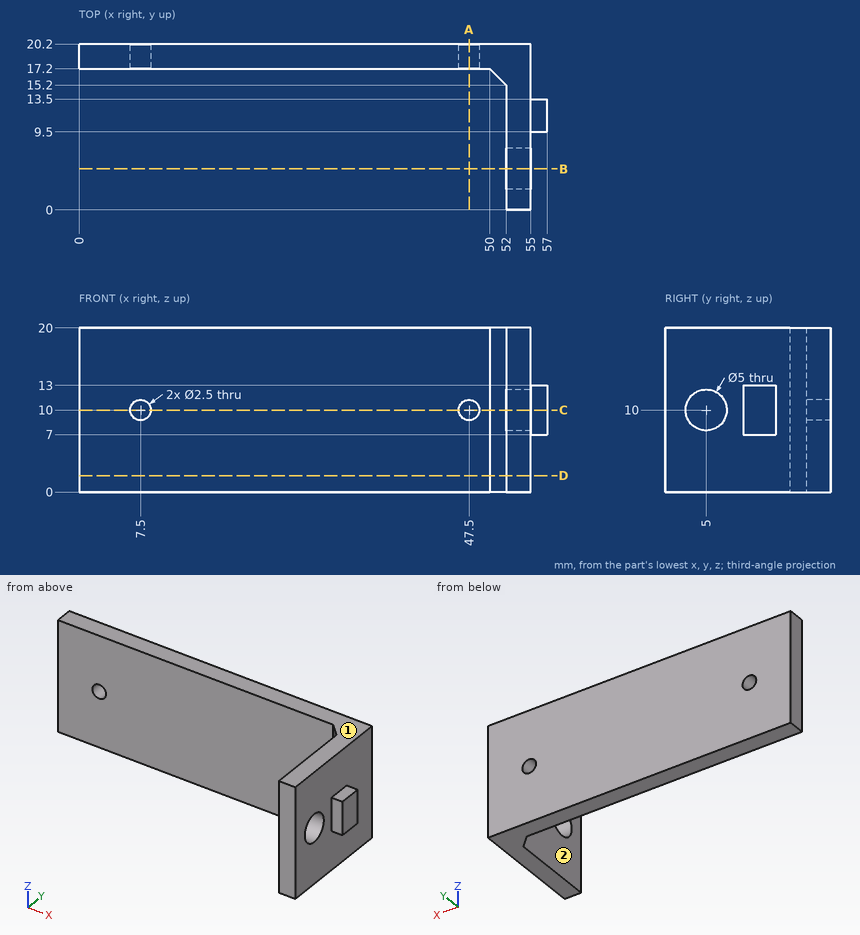
Verification items for this drawing (mm, ordinates from the low corner). A direction names the side the tool comes from. Round coordinates to 2 decimals unless told otherwise and drop trailing zeros. Loops run counter-clockwise (first coordinate to the right, second up) from the corner with the lowest first, then second, coordinate; pieces in that order, holes last. Notation, with made-up numbers: (31.25, 83) -> (78.25, 83) arc R19 cw to (78.25, 111) -> close; hole circle Ø9 at (47, 24.25). An arc over 180 degrees is marked (long way). Answer in a Markdown table with one row per item.
Q1. Go/stop test with flat-tipped pins: P1, Ø3, axis at y = 4.5, z = 5.5, coming from the +X side; P2, Ø0.6, axis at x = 56.5, y = 11.5, coming from the -Z side; P3, Ø0.6, axis at x = 56.5, y = 12.5, coming from the +Z side; P4, Ø1.5, axis at x = 47.5, z = 10, coming from the +Y side. Record where each tip stops, or that it passes through.
Data:
| item | result |
|---|---|
| P1 | stops at x = 55 |
| P2 | stops at z = 7 |
| P3 | stops at z = 13 |
| P4 | passes through |
Q2. Sectioned sample at B-B on y = 5. Enter the section's corners in (x, z), then the cut area to 3 significant figures.
Data:
| item | result |
|---|---|
| outline | (52, 0) -> (55, 0) -> (55, 7.5) -> (52, 7.5) -> close; (52, 12.5) -> (55, 12.5) -> (55, 20) -> (52, 20) -> close |
| area | 45.0 mm^2 |
Q3. Sectioned sample at D-D on z = 2. Enter the section's corners in (x, y), then the cut area to 3 significant figures.
Data:
| item | result |
|---|---|
| outline | (0, 17.2) -> (50, 17.2) -> (52, 15.2) -> (52, 0) -> (55, 0) -> (55, 20.2) -> (0, 20.2) -> close |
| area | 219 mm^2 |
Q4. Set-up check for the marked faces 1 and 2: record each of +Z, -Z, +X, -X, +Y, -Y from which the full face is reachable in a straight line by a thin tool's end or side.
Data:
| item | result |
|---|---|
| face 1 | +Z, +X, -X, +Y, -Y |
| face 2 | +Z, -Z, -X, -Y |
Q5. Sectioned sample at A-A on x = 47.5. Enter the section's corners in (y, z), then the cut area to 3 significant figures.
Data:
| item | result |
|---|---|
| outline | (17.2, 0) -> (20.2, 0) -> (20.2, 8.75) -> (17.2, 8.75) -> close; (17.2, 11.25) -> (20.2, 11.25) -> (20.2, 20) -> (17.2, 20) -> close |
| area | 52.5 mm^2 |
Q6. Thickness scan on L1, parallel to Y at x = 54.05, z = 10; L2, parallel to Z at x = 47.5, y = 18.3; L3, parallel to X at y = 3.5, z = 12.25. Record the ranges inside material, lowest first.
Data:
| item | result |
|---|---|
| L1 | y = 0 to 2.5, 7.5 to 20.2 |
| L2 | z = 0 to 8.75, 11.25 to 20 |
| L3 | x = 52 to 55 |
Q7. Sectioned sample at C-C on z = 10. Enter the section's corners in (x, y), then the cut area to 3 significant figures.
Data:
| item | result |
|---|---|
| outline | (0, 17.2) -> (6.25, 17.2) -> (6.25, 20.2) -> (0, 20.2) -> close; (8.75, 17.2) -> (46.25, 17.2) -> (46.25, 20.2) -> (8.75, 20.2) -> close; (48.75, 17.2) -> (50, 17.2) -> (52, 15.2) -> (52, 7.5) -> (55, 7.5) -> (55, 9.5) -> (57, 9.5) -> (57, 13.5) -> (55, 13.5) -> (55, 20.2) -> (48.75, 20.2) -> close; (52, 0) -> (55, 0) -> (55, 2.5) -> (52, 2.5) -> close |
| area | 197 mm^2 |
